Job drawing, mm, ordinate dimensions from the low corner. One solid piece. A direction names the side the tool comes from. Coordinates: 2 decimals unless noted, no trailing zeros. Order: outer loops, then holes, each group sorted by start corner. A loop starts at its lowest first (then second) coordinate and runs counter-clockwise, first axis right, second up. Notation, with made-up numbers: M 29.25,59.25 L 57.25,59.25 A27 cw 57.25,93.25 Z; hole C 55.25,-2 d10. An arc over 180 degrees is marked long. Write item = value, one per line.
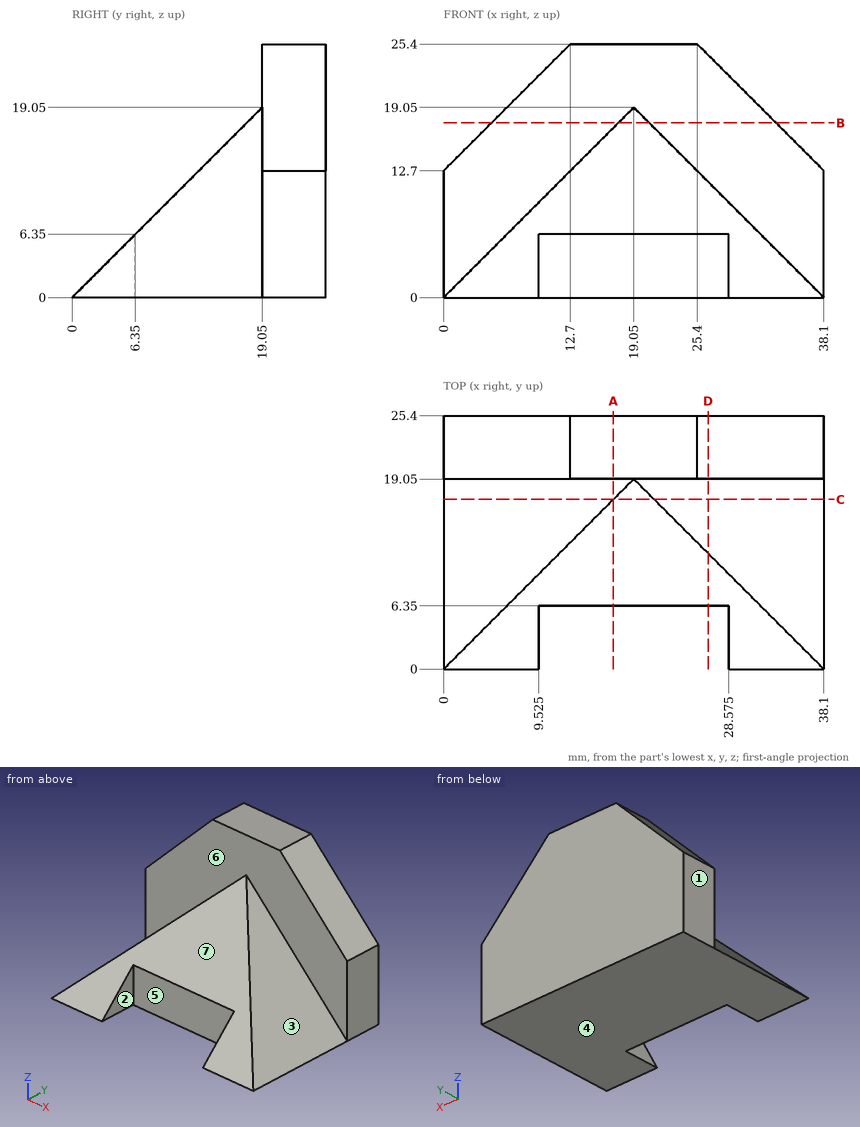
(1) Slice it at C-C, the plane y = 17. Write the cut outline in (x, z).
Evaluation:
outline = M 0,0 L 38.1,0 L 21.1,17 L 17,17 Z
(2) Pin check, flat tips, straight feed: pin 1 Ø7 at (y, z) = (2, 4.5) entering from +X; pin 2 Ø2 at (x, y) = (12, 13.5) entering from +Z; pin 3 Ø7.5 at (x, z) = (16, 17) entering from -Y. Stop position of each tip, or through.
Evaluation:
pin_1 = 37.1
pin_2 = 13
pin_3 = 13.25
(3) Slice it at D-D, the plane x = 26.5. Write the cut outline in (y, z).
Evaluation:
outline = M 6.35,0 L 25.4,0 L 25.4,24.3 L 19.05,24.3 L 19.05,11.6 L 11.6,11.6 L 6.35,6.35 Z
(4) Wall check: line 1 (Y direction, x = 5.5, z = 14.75); line 2 (Y direction, x = 19, z = 3.75); line 3 (Z direction, x = 15, y = 6.5). Give the ranges that are in metal, low to high. Write a range as from..to.
Evaluation:
line_1 = 19.05..25.4
line_2 = 6.35..25.4
line_3 = 0..6.5
(5) Pull direction X, two halves, no side cores. Call the marked faces 1, 2, 3 and 4: +X half, -X half, draft (parallel to the pull), parting line (faces both ways), or undercut.
Evaluation:
face_1 = -X half
face_2 = undercut
face_3 = +X half
face_4 = draft
(6) Slice it at A-A, the plane x = 17. Write the cut outline in (y, z), then the cut area to 3 significant figures.
Evaluation:
outline = M 6.35,0 L 25.4,0 L 25.4,25.4 L 19.05,25.4 L 19.05,17 L 17,17 L 6.35,6.35 Z
area = 320 mm²
(7) Tool access for the marked faces 5, 6 and 7: list every direction of +Z, -Z, +X, -X, +Y, -Y with a clear straight run to the whole face (end or side of a thin tool).
Evaluation:
face_5 = +Z, -Z, -Y
face_6 = +Z, -Y
face_7 = +Z, +X, -X, -Y
(8) Slice it at B-B, the plane z = 17.5. Write the cut outline in (x, y), then the cut area to 3 significant figures.
Evaluation:
outline = M 4.8,19.05 L 17.5,19.05 L 17.5,17.5 L 20.6,17.5 L 20.6,19.05 L 33.3,19.05 L 33.3,25.4 L 4.8,25.4 Z
area = 186 mm²
